from build123d import *

# Parameters (mm, degrees)
CUT_EXTRUDE1_START = -50.8
SKETCH2_R          = 12.7
CUT_EXTRUDE1_DEPTH = 50.8


with BuildPart() as part:
    # Sketch1 → Base-Revolve (revolve)
    with BuildSketch(Plane.XY, mode=Mode.PRIVATE) as base_revolve_sk:
        Polygon((0, 0), (25.4, 0), (25.4, 19.05), (44.45, 19.05), (44.45, 69.85), (25.4, 69.85), (25.4, 82.55), (12.7, 82.55), (12.7, 133.35), (0, 133.35), align=None)
    revolve(base_revolve_sk.sketch.rotate(Axis((0, 0, 0), (0, -1, 0)), 90), axis=Axis((0, 0, 0), (0, -1, 0)))

    # Sketch2 → Cut-Extrude1 (cut)
    with BuildSketch(Plane.XZ.offset(CUT_EXTRUDE1_START)):
        with Locations(Location((0, 0, 0), (0, 0, 90))):
            Circle(SKETCH2_R)
    extrude(amount=CUT_EXTRUDE1_DEPTH, mode=Mode.SUBTRACT)


solid = part.part
Check sheet for the modelled part. Datum: model origin and axes. Units: mm. A direction names the side the tool comes from. Coordinates: 2 decimals unless noted, no trailing zeros. Write each loop counter-clockwise with the first axis right and the second up, starting at its lowest first coordinate (ties: lowest second). Pieces come first, ordered by that corner, then holes. Notation, with made-up numbers: M -23.5,22.5 L 35.5,22.5 A15 cw 35.5,40.5 Z; hole C 65.25,71 d8. An arc over 180 degrees is marked long. Answer as CSV lines item,"result".
Q1. Mould release check, pull along X, two halves, no side actions. Record for faces 1 (the face through (-12, 82.55, 5)), 2 (the face through (-30, 44.8, -32.8)), 3 (the face through (0, 50.8, 0)): released by +X, released by -X, zero draft, split by the parting line, or undercut.
Check result:
face 1,"zero draft"
face 2,"split by the parting line"
face 3,"undercut"
Q2. Cross-section at D-D (y = 98.5). Record the boundary of the cut face in (x, z).
Check result:
outline,"C 0,0 d25.4"
Q3. Cross-section at C-C (y = 47). Record the boundary of the cut face in (x, z).
Check result:
outline,"C 0,0 d88.9; hole C 0,0 d25.4"
Q4. Cross-section at B-B (z = 0). Record the boundary of the cut face in (x, y).
Check result:
outline,"M -44.45,19.05 L -25.4,19.05 L -25.4,0 L -12.7,0 L -12.7,50.8 L 12.7,50.8 L 12.7,0 L 25.4,0 L 25.4,19.05 L 44.45,19.05 L 44.45,69.85 L 25.4,69.85 L 25.4,82.55 L 12.7,82.55 L 12.7,133.35 L -12.7,133.35 L -12.7,82.55 L -25.4,82.55 L -25.4,69.85 L -44.45,69.85 Z"
Q5. Set-up check for faces 4 (the face through (0, 133.35, 0)), 5 (the face through (19, 19.05, -19)), 6 (the face through (19, 69.85, 19)): record each of +Z, -Z, +X, -X, +Y, -Y from which the full face is reachable in a straight line by a thin tool's end or side.
Check result:
face 4,"+Z, -Z, +X, -X, +Y"
face 5,"-Y"
face 6,"+Y"
Q6. Cross-section at A-A (x = 0). Record the boundary of the cut face in (y, z), then the cut area to 3 significant figures.
Check result:
outline,"M 0,-25.4 L 19.05,-25.4 L 19.05,-44.45 L 69.85,-44.45 L 69.85,-25.4 L 82.55,-25.4 L 82.55,-12.7 L 133.35,-12.7 L 133.35,12.7 L 82.55,12.7 L 82.55,25.4 L 69.85,25.4 L 69.85,44.45 L 19.05,44.45 L 19.05,25.4 L 0,25.4 L 0,12.7 L 50.8,12.7 L 50.8,-12.7 L 0,-12.7 Z"
area,"6,130 mm^2"
Q7. Go/stop test with flat-tipped pins: pin 1 (6 mm diameter, centred on x = -32.5, y = 59, fed in from +Z); pin 2 (10 mm diameter, centred on x = -10, y = 91.5, fed in from -Z); pin 3 (12 mm diameter, centred on y = 48.5, z = 33.5, fed in from -X). Record where each tip stops, or that it passes through.
Check result:
pin 1,"z = 33.25"
pin 2,"z = -11.67"
pin 3,"x = -34.92"
Q8. Material ranges on probe 1 along X at (y, z) = (21.5, 0); probe 2 along X at (y, z) = (11, 0); probe 3 along Y at (x, z) = (14.5, -26), recorded low to high. Write a range as from..to.
Check result:
probe 1,"-44.45..-12.7, 12.7..44.45"
probe 2,"-25.4..-12.7, 12.7..25.4"
probe 3,"19.05..69.85"
